For this review, take the finished solid that the model builds, in its own axes (mm). A direction names the side the tool comes from. Coordinates: 2 decimals unless noted, no trailing zeros. Loops run counter-clockwise (first coordinate to the right, second up) from the corner with the lowest first, then second, coordinate; pieces in that order, holes last. Notation, with made-up numbers: (44, 65.25) -> (49, 65.25) arc R22 ccw to (49, 102.25) -> close; hole circle Ø5 at (-5, -8). An arc over 180 degrees is marked (long way). One line per item, written item: value.
from build123d import *

# Parameters (mm, degrees)
F0_W      = 73.406
F0_H      = 28.575
F1_DEPTH  = 14.224
F3_DEPTH  = 28.575
F5_DEPTH  = 127
F9_DEPTH  = 4.7752
F11_DEPTH = 4.7752
F13_DEPTH = 4.7752
F15_DEPTH = 25.4


with BuildPart() as f1:
    # F0 (on Top) → F1 (new body, symmetric)
    with BuildSketch(Plane.XY):
        Rectangle(F0_W, F0_H)
    extrude(amount=F1_DEPTH, both=True)

    # F2 (on face) → F3 (join)
    with BuildSketch(Plane.XY.offset(14.224)):
        Polygon((26.32423571, 7.9375), (-36.703, 7.9375), (-36.703, -2.9845), (-30.353, -2.9845), (-30.353, -7.8105), (26.32423571, -7.8105), (26.32423571, -12.7), (36.703, -12.7), (36.703, 12.7), (26.32423571, 12.7), align=None)
        Polygon((69.4182, 12.7), (36.703, 12.7), (36.703, -12.7), (69.4182, -12.7), (69.4182, 0), align=None)
    extrude(amount=F3_DEPTH)

    # F4 (on face) → F5 (cut)
    with BuildSketch(Plane.XZ.offset(12.7)):
        Polygon((69.4182, 14.224), (69.4182, 42.799), (40.8432, 14.224), align=None)
    extrude(amount=-F5_DEPTH, mode=Mode.SUBTRACT)

    # F6: F1 across plane


with BuildPart() as f1_1:
    add(f1.part)
    add(f1.part.mirror(Plane.XY))

    # F7 (on face) + F8 (on face) → F9 (cut)
    with BuildSketch(Plane.XZ.offset(12.7)):
        Polygon((51.8922, 25.273), (32.893, 25.273), (26.32423571, 25.273), (26.32423571, 14.224), (36.703, 14.224), (40.8432, 14.224), align=None)
    with BuildSketch(Plane.XZ.offset(12.7)):
        Polygon((26.32423571, -14.224), (26.32423571, -25.273), (51.8922, -25.273), (40.8432, -14.224), (36.703, -14.224), align=None)
    extrude(amount=-F9_DEPTH, mode=Mode.SUBTRACT)

    # F10 (on face) → F11 (cut)
    with BuildSketch(Plane(origin=(0, 12.7, 0), x_dir=(-1, 0, 0), z_dir=(0, 1, 0))):
        Polygon((-40.8432, -14.224), (-51.8922, -25.273), (-26.32423571, -25.273), (-26.32423571, -14.224), (-36.703, -14.224), align=None)
    extrude(amount=-F11_DEPTH, mode=Mode.SUBTRACT)

    # F12 (on face) → F13 (cut)
    with BuildSketch(Plane(origin=(0, 12.7, 0), x_dir=(-1, 0, 0), z_dir=(0, 1, 0))):
        Polygon((-26.32423571, 25.273), (-51.8922, 25.273), (-40.8432, 14.224), (-36.703, 14.224), (-26.32423571, 14.224), align=None)
    extrude(amount=-F13_DEPTH, mode=Mode.SUBTRACT)

    # F14 (on face) → F15 (cut)
    with BuildSketch(Plane.XZ.offset(7.8105)):
        with BuildLine():
            Line((17.399, 35.814), (-6.477, 35.814))
            ThreePointArc((-6.477, 35.814), (-12.065, 30.226), (-6.477, 24.638))
            Line((-6.477, 24.638), (17.399, 24.638))
            ThreePointArc((17.399, 24.638), (22.987, 30.226), (17.399, 35.814))
        make_face()
        with BuildLine():
            Line((17.399, -24.638), (-6.477, -24.638))
            ThreePointArc((-6.477, -24.638), (-12.065, -30.226), (-6.477, -35.814))
            Line((-6.477, -35.814), (17.399, -35.814))
            ThreePointArc((17.399, -35.814), (22.987, -30.226), (17.399, -24.638))
        make_face()
    extrude(amount=-F15_DEPTH, mode=Mode.SUBTRACT)


solid = f1_1.part
1. Take a section at D-D, the plane y = -6.5. Give the boundary of the cut face in (x, z), and give its area (3 significant figures).
Return value:
outline: (-36.7, -14.22) -> (-30.35, -14.22) -> (-30.35, -42.8) -> (69.42, -42.8) -> (40.84, -14.22) -> (36.7, -14.22) -> (36.7, 14.22) -> (40.84, 14.22) -> (69.42, 42.8) -> (-30.35, 42.8) -> (-30.35, 14.22) -> (-36.7, 14.22) -> close; hole (-6.48, -35.81) -> (17.4, -35.81) arc R5.59 ccw to (17.4, -24.64) -> (-6.48, -24.64) arc R5.59 ccw to start; hole (-6.48, 24.64) -> (17.4, 24.64) arc R5.59 ccw to (17.4, 35.81) -> (-6.48, 35.81) arc R5.59 ccw to start
area: 6,240 mm2
2. The part is to be moulded in two halves that separate along X. For faces 6 (the flat face through (58.51, -0.18, 31.89)), 7 (the flat face through (27, 0, 42.799)), 8 (the cylindrical face through (-12.064, -0.047, 30.349)), say which applies: pulls with the +X half, pulls with the -X half, needs draft (parallel to the pull), parting line crosses it, or undercut.
Return value:
face 6: pulls with the +X half
face 7: needs draft
face 8: undercut
3. Take a section at C-C, the plane x = 39.5. Give the boundary of the cut face in (y, z), and give its area (3 significant figures).
Return value:
outline: (-12.7, -42.8) -> (12.7, -42.8) -> (12.7, -25.27) -> (7.92, -25.27) -> (7.92, -14.22) -> (-7.92, -14.22) -> (-7.92, -25.27) -> (-12.7, -25.27) -> close; (-12.7, 25.27) -> (-7.92, 25.27) -> (-7.92, 14.22) -> (7.92, 14.22) -> (7.92, 25.27) -> (12.7, 25.27) -> (12.7, 42.8) -> (-12.7, 42.8) -> close
area: 1,240 mm2
4. To check wall thickness, follow probe 1 along Z at (x, y) = (11.5, -5); probe 2 along Z at (x, y) = (30.5, -10); probe 3 along X at (y, z) = (1.5, 12). State the ranges of each line that lie inside material, in increasing order. Write a range as from..to.
Return value:
probe 1: z = -42.8..-35.81, -24.64..24.64, 35.81..42.8
probe 2: z = -42.8..-25.27, -14.22..14.22, 25.27..42.8
probe 3: x = -36.7..36.7
5. Insertion check: pin 1 Ø9 at (x, z) = (38.5, -34.5) entering from -Y; pin 2 Ø2.5 at (y, z) = (-6, 28.5) entering from -X; pin 3 Ø8 at (x, z) = (-15.5, 22.5) entering from -Y. Each pin has a flat end and moves straight along its axis. Give the tip position at first contact, or say it passes through.
Return value:
pin 1: stops at y = -12.7
pin 2: stops at x = -30.35
pin 3: stops at y = -7.81
6. Take a section at A-A, the plane x = 9.5. Give the boundary of the cut face in (y, z).
Return value:
outline: (-14.29, -14.22) -> (-7.81, -14.22) -> (-7.81, -24.64) -> (7.94, -24.64) -> (7.94, -14.22) -> (14.29, -14.22) -> (14.29, 14.22) -> (7.94, 14.22) -> (7.94, 24.64) -> (-7.81, 24.64) -> (-7.81, 14.22) -> (-14.29, 14.22) -> close; (-7.81, -42.8) -> (7.94, -42.8) -> (7.94, -35.81) -> (-7.81, -35.81) -> close; (-7.81, 35.81) -> (7.94, 35.81) -> (7.94, 42.8) -> (-7.81, 42.8) -> close
7. Take a section at B-B, the plane y = 10.75. Give the boundary of the cut face in (x, z).
Return value:
outline: (-36.7, -14.22) -> (36.7, -14.22) -> (36.7, 14.22) -> (-36.7, 14.22) -> close; (26.32, -42.8) -> (69.42, -42.8) -> (51.89, -25.27) -> (26.32, -25.27) -> close; (26.32, 25.27) -> (51.89, 25.27) -> (69.42, 42.8) -> (26.32, 42.8) -> close
8. For faces 1 (the flat face through (58.51, -0.18, -31.89)), 2 (the flat face through (43, 12.7, -34)), 3 (the flat face through (5, 0, -35.814)), 4 (the flat face through (-2, -7.81, 22)), 5 (the flat face through (26.324, 10, 34)), list the 3-axis set-ups (+Z, -Z, +X, -X, +Y, -Y) from which the entire face can be reached by the end or side of a thin tool; tool diameter is ignored.
Return value:
face 1: +X, +Y, -Y
face 2: -Z, +X, -X, +Y
face 3: +Y, -Y
face 4: +Z, -X, -Y
face 5: +Z, -X, +Y
